Build history of the part. All positions in model axes, mm. Coordinates: 2 decimals unless noted, no trailing zeros. Write each loop counter-clockwise with the first axis right and the second up, starting at its lowest first coordinate (ties: lowest second). Pieces come first, ordered by that corner, then holes. Notation, with made-up numbers: M -26.5,75 L -19.5,75 A26 ccw -19.5,89 Z; hole C -26.5,26.5 d10. An arc over 180 degrees is marked long. Use CSV: the item, a comma, the result in double quotes. Start each with the question number.
Autodesk Inventor part; units mm, degrees
ref_plane "YZ Plane" through (0, 0, 0) normal (1, 0, 0) x (0, 1, 0)
ref_plane "XZ Plane" through (0, 0, 0) normal (0, 1, 0) x (-1, 0, 0)
ref_plane "XY Plane" through (0, 0, 0) normal (0, 0, 1) x (1, 0, 0)
sketch "Sketch1" plane through (0, 0, 0) normal (0, 0, 1) x (1, 0, 0)
  line L0 (-60, -120) -> (60, -120)
  line L1 (60, -120) -> (60, 120)
  line L2 (60, 120) -> (-60, 120)
  line L3 (-60, 120) -> (-60, -120)
  line L4 (-60, -120) -> (60, 120) construction
  line L5 (60, -120) -> (-60, 120) construction
  line L6 (40, -100) -> (-40, -100)
  line L7 (-40, -100) -> (-40, 100)
  line L8 (-40, 100) -> (40, 100)
  line L9 (40, 100) -> (40, -100)
  line L10 (40, -100) -> (-40, 100) construction
  line L11 (-40, -100) -> (40, 100) construction
  point P0 (0, 0)
  dimension "d172" = 80
  dimension "d180" = 20
  dimension "d181" = 20
  dimension "d182" = 200
extrude "Plate5" add sketch "Sketch1" along normal blind 3
sketch "Sketch9" plane through (0, 0, 3) normal (0, 0, 1) x (1, 0, 0)
  circle A0 centre (53, -113) radius 3
  line L0 (53, 113) -> (-53, 113) construction
  line L1 (-53, 113) -> (-53, -113) construction
  line L2 (-53, -113) -> (53, -113) construction
  line L3 (53, -113) -> (53, 113) construction
  line L4 (53, 113) -> (-53, -113) construction
  line L5 (-53, 113) -> (53, -113) construction
  circle A1 centre (-53, -113) radius 3
  circle A2 centre (53, 113) radius 3
  circle A3 centre (-53, 113) radius 3
  line L6 (-40, -100) -> (-40, 100)
  line L7 (-40, 100) -> (40, 100)
  line L8 (40, 100) -> (40, -100)
  line L9 (40, -100) -> (-40, -100)
  line L10 (60, -120) -> (-60, -120)
  line L11 (60, 120) -> (60, -120)
  line L12 (-60, 120) -> (60, 120)
  line L13 (-60, -120) -> (-60, 120)
  circle A4 centre (-53, 0) radius 3
  circle A5 centre (53, 0) radius 3
  point P0 (0, 0)
  dimension "d174" = 6
  dimension "d183" = 7
  dimension "d184" = 7
extrude "Cut2" cut sketch "Sketch9" against normal blind 3 contours A0 | A1 | A2 | A3 | A4 | A5
fillet "Corner Round1" radius 6 4 edges at (60, 120, 1.5) (-60, 120, 1.5) (-60, -120, 1.5) (60, -120, 1.5)
properties part number "TKS 3521 BOTTOM FDS Diam way flange 1" material "Stainless Steel"
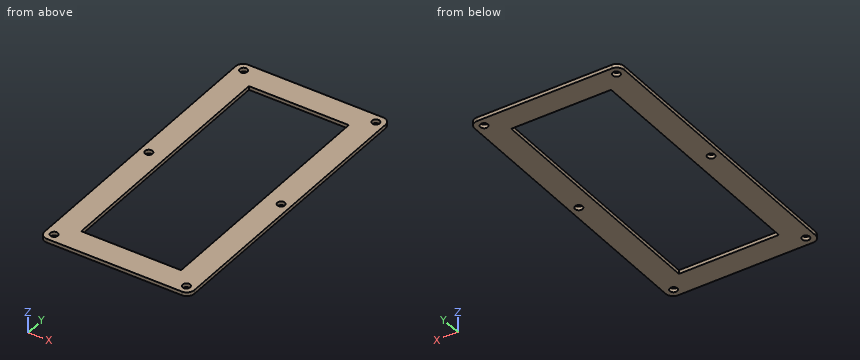
1. Slice it at A-A (x = 26). List the corners of the cut face in (y, z), and give its area (3 significant figures).
2. Slice it at C-C (z = 0.8). List the corners of the cut face in (x, y), and give its area (3 significant figures).
3. Drill centre lines: line 1 along Y through (x, z) = (53, 0.95); line 2 along X through (y, z) = (-18.5, 0.35); line 3 along Y through (x, z) = (21, 0.85). Where is each one in solid material? Low to high. Write a range as from..to.
4. Slice it at B-B (y = 0). List the corners of the cut face in (x, z).
Established:
1,outline,"M -120,0 L -100,0 L -100,3 L -120,3 Z; M 100,0 L 120,0 L 120,3 L 100,3 Z"
1,area,"120 mm2"
2,outline,"M -60,-114 A6 ccw -54,-120 L 54,-120 A6 ccw 60,-114 L 60,114 A6 ccw 54,120 L -54,120 A6 ccw -60,114 Z; hole C -53,-113 d6; hole C -53,0 d6; hole C -53,113 d6; hole M -40,-100 L 40,-100 L 40,100 L -40,100 Z; hole C 53,-113 d6; hole C 53,0 d6; hole C 53,113 d6"
2,area,"12,600 mm2"
3,line 1,"y = -120..-116, -110..-3, 3..110, 116..120"
3,line 2,"x = -60..-40, 40..60"
3,line 3,"y = -120..-100, 100..120"
4,outline,"M -60,0 L -56,0 L -56,3 L -60,3 Z; M -50,0 L -40,0 L -40,3 L -50,3 Z; M 40,0 L 50,0 L 50,3 L 40,3 Z; M 56,0 L 60,0 L 60,3 L 56,3 Z"
